```python
from build123d import *

# Parameters (mm, degrees)
SKETCH1_W            = 533.4
SKETCH1_H            = 622.3
BOSS_EXTRUDE1_DEPTH  = 3.175
CUT_EXTRUDE1_DEPTH   = 4.175
LPATTERN1_COUNT      = 2
LPATTERN1_PITCH      = 520.7
LPATTERN1_COUNT_DIR2 = 2
LPATTERN1_PITCH_DIR2 = 495.3
SKETCH5_W            = 215.9
SKETCH5_H            = 82.55
CUT_EXTRUDE3_DEPTH   = 4.175
SKETCH6_W            = 215.9
SKETCH6_H            = 34.925
CUT_EXTRUDE4_DEPTH   = 4.175


with BuildPart() as part:
    # Sketch1 → Boss-Extrude1 (new body)
    with BuildSketch(Plane.XY):
        with Locations((266.7, 311.15)):
            Rectangle(SKETCH1_W, SKETCH1_H)
    extrude(amount=BOSS_EXTRUDE1_DEPTH)

    # Sketch2 → Cut-Extrude1 (cut, through all)
    with BuildSketch(Plane.XY.offset(3.175)):
        with BuildLine():
            Line((14.2875, 574.8782), (23.8125, 574.8782))
            ThreePointArc((23.8125, 574.8782), (27.1907, 571.5), (23.8125, 568.1218))
            Line((23.8125, 568.1218), (14.2875, 568.1218))
            ThreePointArc((14.2875, 568.1218), (10.9093, 571.5), (14.2875, 574.8782))
        make_face()
    cut_extrude1 = extrude(amount=-CUT_EXTRUDE1_DEPTH, mode=Mode.SUBTRACT)

    # LPattern1: Cut-Extrude1 2 × 2
    with Locations(*[(j * LPATTERN1_PITCH_DIR2, -i * LPATTERN1_PITCH, 0) for i in range(LPATTERN1_COUNT) for j in range(LPATTERN1_COUNT_DIR2) if (i, j) != (0, 0)]):
        add(cut_extrude1, mode=Mode.SUBTRACT)

    # Sketch5 → Cut-Extrude3 (cut, through all)
    with BuildSketch(Plane(origin=(0, 0, 0), x_dir=(-1, 0, 0), z_dir=(0, 0, -1))):
        with Locations((-266.7, 494.422045059)):
            Rectangle(SKETCH5_W, SKETCH5_H)
    extrude(amount=-CUT_EXTRUDE3_DEPTH, mode=Mode.SUBTRACT)

    # Sketch6 → Cut-Extrude4 (cut, through all)
    with BuildSketch(Plane(origin=(0, 0, 0), x_dir=(-1, 0, 0), z_dir=(0, 0, -1))):
        with Locations((-266.7, 17.4625)):
            Rectangle(SKETCH6_W, SKETCH6_H)
    extrude(amount=-CUT_EXTRUDE4_DEPTH, mode=Mode.SUBTRACT)


solid = part.part
```
Work out the finished part from the listing and answer in its coordinate system (mm). Give positions to 0.01 mm unless a question says otherwise; leave off trailing zeros. Order: outer loops, then holes, each group sorted by start corner. A loop starts at its lowest first (then second) coordinate and runs counter-clockwise, first axis right, second up.
1. Straight lines are drawn through the part: L1, parallel to X at y = 501, z = 0.5; L2, parallel to Y at x = 25.5, z = 0.25; L3, parallel to Y at x = 230.5, z = 0.65 (3 decimals). For each, find the intervals that lie inside material, in ascending order.
Result sheet:
L1: x = 0 to 158.75, 374.65 to 533.4
L2: y = 0 to 47.87, 53.73 to 568.57, 574.43 to 622.3
L3: y = 34.925 to 453.147, 535.697 to 622.3
2. Section B-B, the plane x = 271.5 is taken. Determine the outline of the cut face in (y, z) (3 decimals), and give its area (3 significant figures).
Result sheet:
outline: (34.925, 0) - (453.147, 0) - (453.147, 3.175) - (34.925, 3.175) - close; (535.697, 0) - (622.3, 0) - (622.3, 3.175) - (535.697, 3.175) - close
area: 1,600 mm2
3. Section A-A, the plane z = 1.2 is taken. Give the number of separate pieces and of enclosed holes in the cut face, and give its area (3 significant figures).
Result sheet:
separate pieces: 1
enclosed holes: 5
area: 306,000 mm2
4. This flat-tipped pin is pushed along its axis until it touches: P1, Ø12, axis at x = 266.5, y = 333.5, coming from the -Z side. Where does it stop, or does it pass through?
Result sheet:
P1: stops at z = 0
